from build123d import *

# Parameters (mm, degrees)
BASES_R             = 6.35
BASE_DEPTH          = 5.4
TOPBORES_R          = 1.75
TOP_BORE_DEPTH      = 11.478788098
HORN_START          = -2.5
HORN_HALF_DEPTH     = 2.5
HORNATTACHS_R       = 1.65
HORN_ATTACH_DEPTH   = 21.913031822
HOLDINGSHAFTS_R     = 6.35
HOLDINGSHAFTS_R_2   = 4.25
HOLDING_SHAFT_DEPTH = 2.9
SKETCH3_R           = 3.025
CUT_EXTRUDE2_DEPTH  = 2.9


with BuildPart() as part:
    # BaseS → BASE (new body)
    with BuildSketch(Plane(origin=(0, 0, 0), x_dir=(1, 0, 0), z_dir=(0, 1, 0))):
        with Locations(Location((0, 0, 0), (0, 0, 90))):
            Circle(BASES_R)
    extrude(amount=BASE_DEPTH)

    # TopBoreS → TOP BORE (cut, through all)
    with BuildSketch(Plane(origin=(0, 5.4, 0), x_dir=(1, 0, 0), z_dir=(0, 1, 0))):
        with Locations(Location((0, 0, 0), (0, 0, 270))):
            Circle(TOPBORES_R)
    extrude(amount=-TOP_BORE_DEPTH, mode=Mode.SUBTRACT)

    # HornHalfS → HORN HALF (add)
    with BuildSketch(Plane(origin=(0, 5.4, 0), x_dir=(1, 0, 0), z_dir=(0, 1, 0)).offset(HORN_START)):
        with BuildLine():
            Line((-3.102144422, 16.57699176), (-5.450702003, 3.257659846))
            ThreePointArc((-5.450702003, 3.257659846), (0, 6.35), (5.450702003, 3.257659846))
            Line((5.450702003, 3.257659846), (3.102144422, 16.57699176))
            ThreePointArc((3.102144422, 16.57699176), (0, 19.18), (-3.102144422, 16.57699176))
        make_face()
    extrude(amount=HORN_HALF_DEPTH)

    # HornAttachS → HORN ATTACH (cut, through all)
    with BuildSketch(Plane(origin=(0, 5.4, 0), x_dir=(1, 0, 0), z_dir=(0, 1, 0))):
        with Locations(Location((0, 16.03, 0), (0, 0, 270))):
            Circle(HORNATTACHS_R)
    extrude(amount=-HORN_ATTACH_DEPTH, mode=Mode.SUBTRACT)

    # HoldingShaftS → HOLDING SHAFT (cut)
    with BuildSketch(Plane.XZ):
        Circle(HOLDINGSHAFTS_R)
        with Locations(Location((0, 0, 0), (0, 0, 270))):
            Circle(HOLDINGSHAFTS_R_2, mode=Mode.SUBTRACT)
    extrude(amount=-HOLDING_SHAFT_DEPTH, mode=Mode.SUBTRACT)

    # Sketch3 → Cut-Extrude2 (cut)
    with BuildSketch(Plane.XZ):
        with Locations(Location((0, 0, 0), (0, 0, 270))):
            Circle(SKETCH3_R)
    extrude(amount=-CUT_EXTRUDE2_DEPTH, mode=Mode.SUBTRACT)


solid = part.part
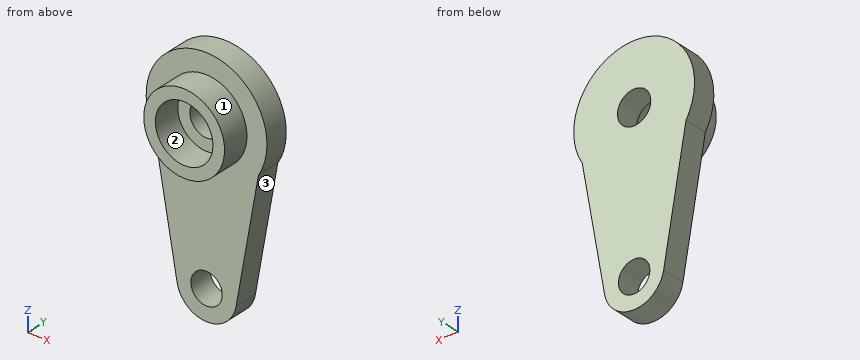
Build history of the part. All positions in model axes, mm. Face numbers are marked on the shaded views. Round coordinates to 2 decimals unless told otherwise and drop trailing zeros. Write each loop counter-clockwise with the first axis right and the second up, starting at its lowest first coordinate (ties: lowest second). Pieces come first, ordered by that corner, then holes. Notation, with made-up numbers: (88, -6) - (130, -6) arc R21 cw to (130, 23) - close; hole circle Ø10 at (-30, 12). An arc over 180 degrees is marked (long way). Use CSV: the item, a comma, the result in double quotes.
(1) Wall check: line 1 (X direction, y = 0.65, z = 0) (3 decimals); line 2 (X direction, y = 3.5, z = 0); line 3 (Y direction, x = -2.75, z = 4.5). Give the ranges that are in metal, low to high.
Response:
line 1,"-4.25 to -3.025, 3.025 to 4.25"
line 2,"-6.35 to -1.75, 1.75 to 6.35"
line 3,"2.9 to 5.4"
(2) Band-saw the part on B-B (z = 0). Write the cut outline in (x, y) (3 decimals), plus the area to 3 significant figures.
Response:
outline,"(-6.35, 2.9) - (-4.25, 2.9) - (-4.25, 0) - (-3.025, 0) - (-3.025, 2.9) - (-1.75, 2.9) - (-1.75, 5.4) - (-6.35, 5.4) - close; (1.75, 2.9) - (3.025, 2.9) - (3.025, 0) - (4.25, 0) - (4.25, 2.9) - (6.35, 2.9) - (6.35, 5.4) - (1.75, 5.4) - close"
area,"30.1 mm²"
(3) Band-saw the part on A-A (x = 0). Write the cut outline in (y, z) (3 decimals), plus the area to 3 significant figures.
Response:
outline,"(0, -4.25) - (2.9, -4.25) - (2.9, -14.38) - (5.4, -14.38) - (5.4, -1.75) - (2.9, -1.75) - (2.9, -3.025) - (0, -3.025) - close; (0, 3.025) - (2.9, 3.025) - (2.9, 1.75) - (5.4, 1.75) - (5.4, 6.35) - (2.9, 6.35) - (2.9, 4.25) - (0, 4.25) - close; (2.9, -19.18) - (5.4, -19.18) - (5.4, -17.68) - (2.9, -17.68) - close"
area,"53.9 mm²"
(4) Pin check, flat tips, straight feed: P1, Ø6.5, axis at x = 1, z = -12, coming from the -Y side; P2, Ø7, axis at x = 0, z = 0, coming from the +Y side; P3, Ø1.5, axis at y = 1, z = -8.5, coming from the +X side. Stop position of each tip, or through.
Response:
P1,"y = 2.9"
P2,"y = 5.4"
P3,"through"
(5) Band-saw the part on C-C (y = 3.15). Write the cut outline in (x, z).
Response:
outline,"(-5.45, -3.26) - (-3.1, -16.58) arc R3.15 ccw to (3.1, -16.58) - (5.45, -3.26) arc R6.35 ccw (long way) to start; hole circle Ø3.5 at (0, 0); hole circle Ø3.3 at (0, -16.03)"
(6) Band-saw the part on D-D (y = 1.7). Write the cut outline in (x, z) (3 decimals), plus the area to 3 significant figures.
Response:
outline,"circle Ø8.5 at (0, 0); hole circle Ø6.05 at (0, 0)"
area,"28.0 mm²"
(7) Mould opens along X. For the marked faces 1, 2 and 3 say: pulls with the +X half, pulls with the -X half, needs draft (parallel to the pull), parting line crosses it, or undercut.
Response:
face 1,"parting line crosses it"
face 2,"undercut"
face 3,"pulls with the +X half"
